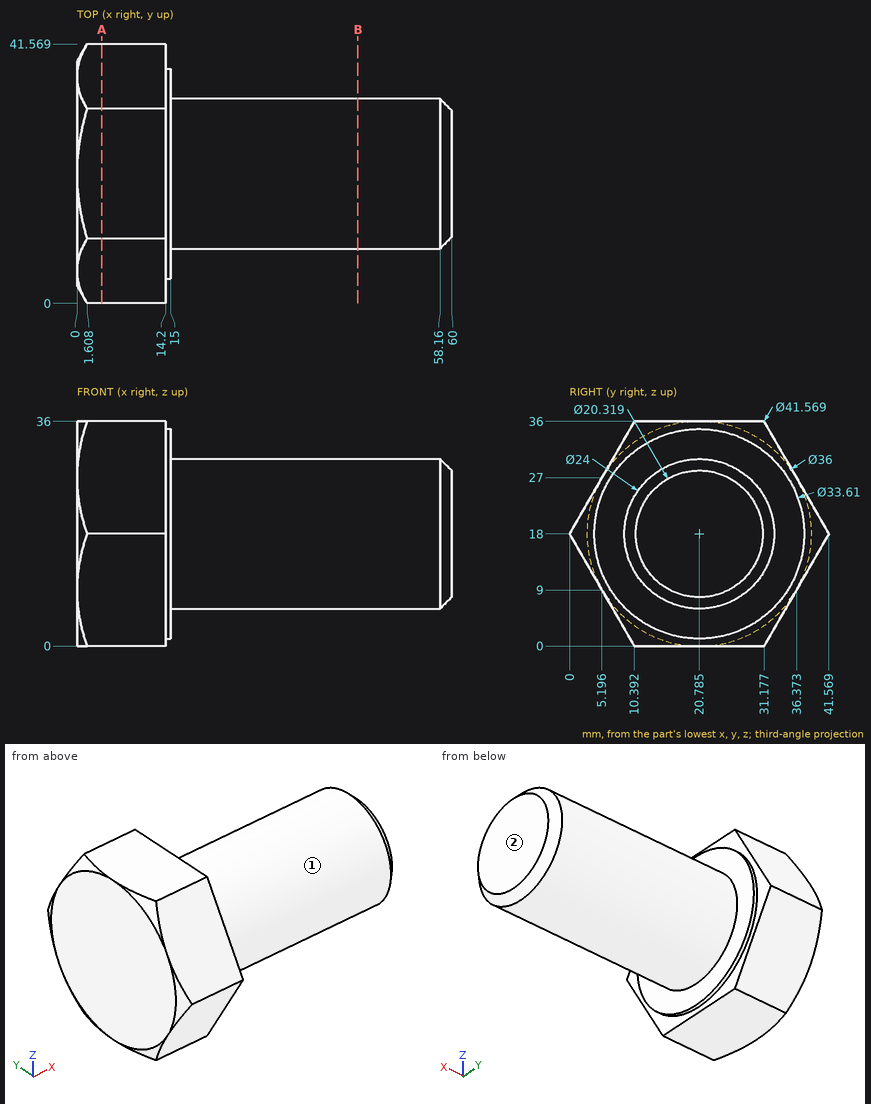
Geometry: see drawing. Coordinates: mm, zero at the bounding-box minimum. A direction names the side the tool comes from. Round coordinates to 2 decimals unless told otherwise and drop trailing zeros. Loops run counter-clockwise (first coordinate to the right, second up) from the corner with the lowest first, then second, coordinate; pieces in that order, holes last. Notation, with made-up numbers: M 2,-3 L 48,-3 A33 cw 48,35 Z; hole C 83,74 d9. An arc over 180 degrees is marked long. Use a Markdown table: item, result. Add a question column.
1. Line query: line 1 (X direction, y = 37, z = 15); line 2 (X direction, y = 8, z = 7); line 3 (Y direction, x = 36, z = 15.5). Output: solid intervals per line, ascending.
2. Section query A-A on x = 4. Return the cut outline in (y, z), then the cut area to 3 significant figures.
3. Contact query for flat-ended pins moving along their axis: P1, Ø2, axis at x = 50, z = 28, coming from the +Y side; P2, Ø3, axis at x = 39, z = 15.5, coming from the +Y side; P3, Ø4, axis at x = 27.5, z = 16.5, coming from the -Y side (1 decimal); P4, Ø5, axis at x = 51.5, y = 36.5, coming from the -Z side. Output: stop coordinate, or through.
4. Reachability of the marked faces 1 and 2 from +Z, -Z, +X, -X, +Y, -Y: full face, straight path, thin tool, end or side. Return the list, or none.
5. Section query B-B on x = 45. Return the cut outline in (y, z) (1 decimal).
Reported:
| question | item | result |
|---|---|---|
| 1 | line 1 | x = 0 to 15 |
| 1 | line 2 | x = 0 to 14.2 |
| 1 | line 3 | y = 9.05 to 32.52 |
| 2 | outline | M 0,18 L 10.39,0 L 31.18,0 L 41.57,18 L 31.18,36 L 10.39,36 Z |
| 2 | area | 1,120 mm² |
| 3 | P1 | stops at y = 28.72 |
| 3 | P2 | stops at y = 32.74 |
| 3 | P3 | stops at y = 8.8 |
| 3 | P4 | passes through |
| 4 | face 1 | +X |
| 4 | face 2 | +Z, -Z, +X, +Y, -Y |
| 5 | outline | C 20.8,18 d24 |
